Build history of the part. All positions in model axes, mm. A direction names the side the tool comes from. Coordinates: 2 decimals unless noted, no trailing zeros. Loops run counter-clockwise (first coordinate to the right, second up) from the corner with the lowest first, then second, coordinate; pieces in that order, holes last. Notation, with made-up numbers: (88.5, 65.5) - (133.5, 65.5) arc R30 cw to (133.5, 102.5) - close; hole circle Ø3 at (76, -7.75). An arc over 180 degrees is marked (long way). One line per item, written item: value.
```python
from build123d import *

# Parameters (mm, degrees)
SKETCH_R        = 2
PAD_DEPTH       = 5
SKETCH001_R     = 13
PAD001_DEPTH    = 8
SKETCH002_R     = 8
POCKET_DEPTH    = 16.001
SKETCH003_W     = 34.242641
SKETCH003_H     = 4
POCKET001_DEPTH = 48.644028
SKETCH004_R     = 11.4
POCKET002_DEPTH = 11
CHAMFER_SIZE    = 3.2


with BuildPart() as part:
    # Sketch → Pad (new body)
    with BuildSketch(Plane.XY):
        with BuildLine():
            Line((1.414214, 0), (49.84062, 0))
            ThreePointArc((49.84062, 0), (51.688379, 1.234633), (51.254834, 3.414214))
            Line((51.254834, 3.414214), (27.041631, 27.627417))
            ThreePointArc((27.041631, 27.627417), (25.627417, 28.213203), (24.213203, 27.627417))
            Line((0, 3.414214), (24.213203, 27.627417))
            ThreePointArc((0, 3.414214), (-0.433546, 1.234633), (1.414214, 0))
        make_face()
        with Locations((4.414214, 3.25)):
            Circle(SKETCH_R, mode=Mode.SUBTRACT)
        with Locations((46.84062, 3.25)):
            Circle(SKETCH_R, mode=Mode.SUBTRACT)
        with Locations((25.627417, 24.463203)):
            Circle(SKETCH_R, mode=Mode.SUBTRACT)
    extrude(amount=PAD_DEPTH)

    # Sketch001 (on Face10 of Pad) → Pad001 (join, symmetric)
    with BuildSketch(Plane(origin=(0, 0, 0), x_dir=(1, 0, 0), z_dir=(0, 0, -1))):
        with Locations((25.627417, 0.536797)):
            Circle(SKETCH001_R)
    extrude(amount=PAD001_DEPTH, both=True)

    # Sketch002 (on Face15 of Pad001) → Pocket (cut, through all)
    with BuildSketch(Plane(origin=(0, 0, -8), x_dir=(1, 0, 0), z_dir=(0, 0, -1))):
        with Locations((25.627417, 0.536797)):
            Circle(SKETCH002_R)
    extrude(amount=-POCKET_DEPTH, mode=Mode.SUBTRACT)

    # Sketch003 (on Face8 of Pocket) → Pocket001 (cut, through all)
    with BuildSketch(Plane(origin=(27.334524, 27.334524, 0), x_dir=(-0.707107, 0.707107, 0), z_dir=(0.707107, 0.707107, 0))):
        with Locations((-16.707106, 7)):
            Rectangle(SKETCH003_W, SKETCH003_H)
    extrude(amount=-POCKET001_DEPTH, mode=Mode.SUBTRACT)

    # Sketch004 (on Face6 of Pocket001) → Pocket002 (cut)
    with BuildSketch(Plane.XY.offset(5)):
        with Locations((25.627417, -0.536797)):
            Circle(SKETCH004_R)
    extrude(amount=-POCKET002_DEPTH, mode=Mode.SUBTRACT)

    # Chamfer
    chamfer_edges = [part.edges().sort_by_distance(p)[0] for p in [
        (14.227417, -0.536797, -6),
    ]]
    chamfer(chamfer_edges, length=CHAMFER_SIZE)


solid = part.part
```
Item 1: Pull direction X, two halves, no side cores. Call faces 4 (the face through (39.32, 15.35, 2.46)), 5 (the face through (29, 11, 5)), 6 (the face through (6.26, 2.48, 2.46)): released by +X, released by -X, zero draft, split by the parting line, or undercut.
Check result:
face 4: released by +X
face 5: zero draft
face 6: undercut
Item 2: Cut at A-A, the plane z = 4.25. Write the cut outline in (x, y), then the cut area to 3 significant figures.
Check result:
outline: (0, 3.41) arc R2 ccw to (1.41, 0) - (12.64, 0) arc R13 ccw (long way) to (38.62, 0) - (49.84, 0) arc R2 ccw to (51.25, 3.41) - (27.04, 27.63) arc R2 ccw to (24.21, 27.63) - close; hole circle Ø4 at (4.41, 3.25); hole circle Ø22.8 at (25.63, -0.54); hole circle Ø4 at (25.63, 24.46); hole circle Ø4 at (46.84, 3.25)
area: 666 mm^2
Item 3: Cut at C-C, the plane y = 2. Give the number of separate pieces and of enclosed holes in the cut face, then the cut area to 3 significant figures.
Check result:
separate pieces: 4
enclosed holes: 0
area: 171 mm^2
Item 4: Drop flat-ended pins along their axis: P1, Ø13, axis at x = 24, y = -3.5, coming from the +Z side; P2, Ø5, axis at x = 34.5, z = -6, coming from the +Y side; P3, Ø1.5, axis at x = 5.5, z = 2.5, coming from the -Y side. Give the stop position or say it passes through.
Check result:
P1: stops at z = -4.32
P2: stops at y = 10.79
P3: stops at y = 0
Item 5: Probe probe 1 along X at (y, z) = (-1, 0.25); probe 2 along Z at (x, y) = (27, 15.5); probe 3 along X at (y, z) = (-2.5, -0.5). List the from-to ranges inside material, lowest first. Write a range as from..to.
Check result:
probe 1: x = 12.64..14.24, 37.02..38.62
probe 2: z = 0..5
probe 3: x = 12.78..14.4, 36.86..38.48
Item 6: Tool access for faces 1 (the face through (25, 14, 0)), 2 (the face through (44, 0, 2)), 3 (the face through (23.935, -13.426, -3.035)): list every direction of +Z, -Z, +X, -X, +Y, -Y with a clear straight run to the whole face (end or side of a thin tool).
Check result:
face 1: -Z, +Y
face 2: +Z, -Z, +X, -Y
face 3: -Z
Item 7: Cut at D-D, the plane x = 12. Write the cut outline in (y, z).
Check result:
outline: (0, 0) - (15.41, 0) - (15.41, 5) - (0, 5) - close
Item 8: Cut at B-B, the plane x = 48. Write the cut outline in (y, z).
Check result:
outline: (0, 0) - (1.62, 0) - (1.62, 5) - (0, 5) - close; (4.88, 0) - (6.67, 0) - (6.67, 5) - (4.88, 5) - close
